Geometry check sheet. Reference: drawing and pictorial views, mm from the part's lowest x, y, z. A direction names the side the tool comes from. Coordinates: 2 decimals unless noted, no trailing zeros. Write each loop counter-clockwise with the first axis right and the second up, starting at its lowest first coordinate (ties: lowest second). Pieces come first, ordered by that corner, then holes. Notation, with made-up numbers: (39.25, -39) -> (82.25, -39) arc R26 cw to (82.25, -6) -> close; hole circle Ø9 at (25, -28.5). An arc over 180 degrees is marked (long way). Put each result on its own line as item: value.
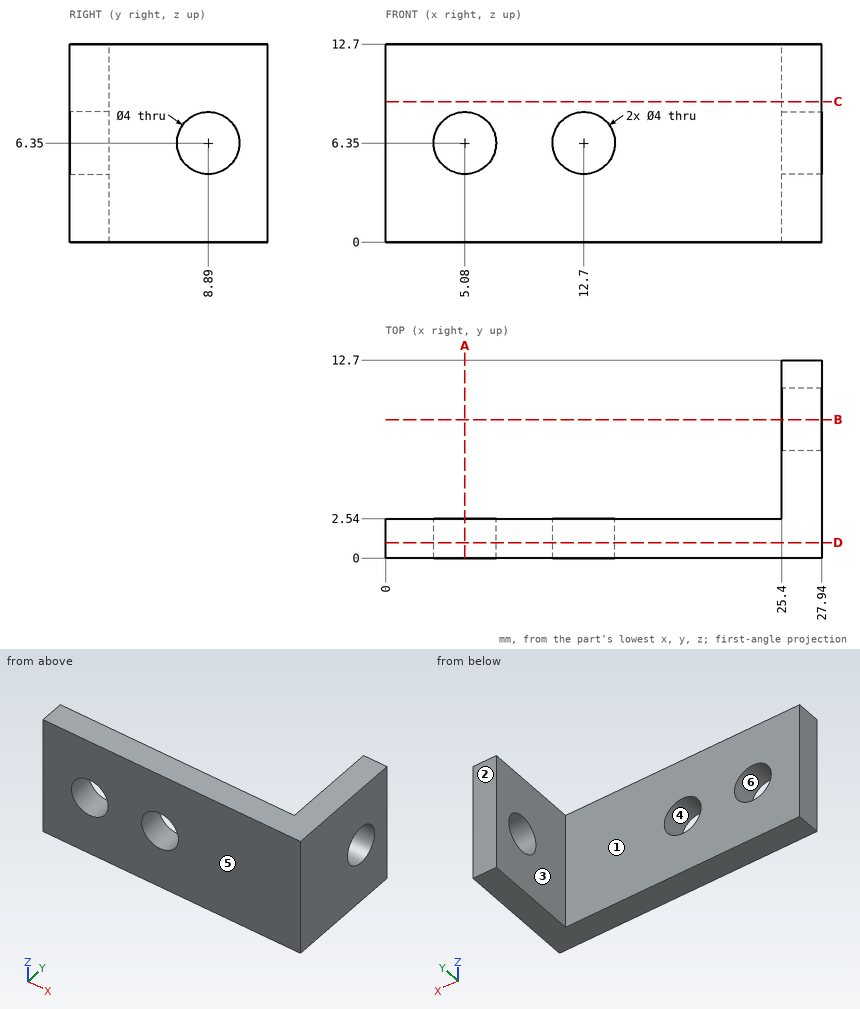
Q1. Material ranges on line 1 along X through (y, z) = (1.45, 6.35); line 2 along X through (y, z) = (2, 5); line 3 along Y through (x, z) = (16, 6.25), recorded low to high.
Recorded:
line 1: x = 0 to 3.08, 7.08 to 10.7, 14.7 to 27.94
line 2: x = 0 to 3.6, 6.56 to 11.22, 14.18 to 27.94
line 3: y = 0 to 2.54
Q2. Cross-section at B-B (y = 8.89). Record the cut outline in (x, z).
Recorded:
outline: (25.4, 0) -> (27.94, 0) -> (27.94, 4.35) -> (25.4, 4.35) -> close; (25.4, 8.35) -> (27.94, 8.35) -> (27.94, 12.7) -> (25.4, 12.7) -> close
Q3. Cross-section at D-D (y = 1). Record the cut outline in (x, z).
Recorded:
outline: (0, 0) -> (27.94, 0) -> (27.94, 12.7) -> (0, 12.7) -> close; hole circle Ø4 at (5.08, 6.35); hole circle Ø4 at (12.7, 6.35)
Q4. Cross-section at A-A (x = 5.08). Record the cut outline in (y, z).
Recorded:
outline: (0, 0) -> (2.54, 0) -> (2.54, 4.35) -> (0, 4.35) -> close; (0, 8.35) -> (2.54, 8.35) -> (2.54, 12.7) -> (0, 12.7) -> close
Q5. Depth check by flat-ended pin: P1, Ø3, axis at y = 8.5, z = 5, coming from the -X side; P2, Ø2, axis at x = 23.5, z = 11, coming from the +Y side. Enter the tip coordinate at first touch or a pass-through.
Recorded:
P1: stops at x = 25.4
P2: stops at y = 2.54
Q6. Cross-section at C-C (z = 9). Record the cut outline in (x, y), plus the area to 3 significant figures.
Recorded:
outline: (0, 0) -> (27.94, 0) -> (27.94, 12.7) -> (25.4, 12.7) -> (25.4, 2.54) -> (0, 2.54) -> close
area: 96.8 mm2
Q7. Tool access check on the marked faces 1 and 2. Record the directions out of +Z, -Z, +X, -X, +Y, -Y that give a thin tool (end or side, any length) a straight path to the whole face; none if there is none.
Recorded:
face 1: +Z, -Z, -X, +Y
face 2: +Z, -Z, +X, -X, +Y
Q8. Mould release check, pull along X, two halves, no side actions. Record for the marked faces 3, 4, 5 and 6: released by +X, released by -X, zero draft, split by the parting line, or undercut.
Recorded:
face 3: released by -X
face 4: undercut
face 5: zero draft
face 6: undercut
